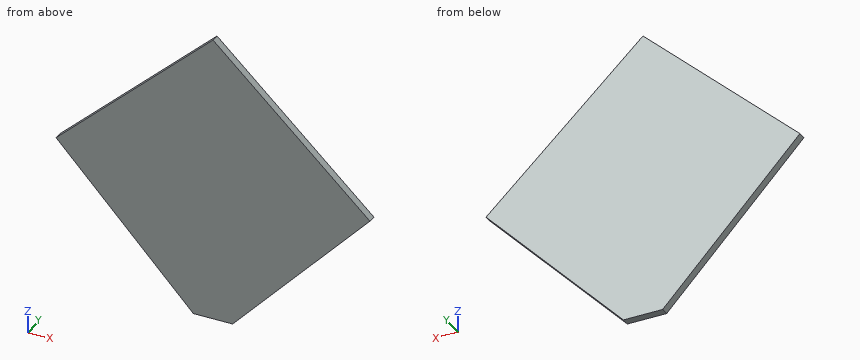
```python
from build123d import *

# Parameters (mm, degrees)
F1_DEPTH = 1


with BuildPart() as f1:
    # F0 (on Front) → F1 (new body)
    with BuildSketch(Plane.XZ):
        Polygon((-2.5, 0), (0, 0), (0, 18.5), (-20, 18.5), align=None)
        Polygon((0, 18.5), (0, 0), (2.5, 0), (20, 18.5), align=None)
        Polygon((-20, 18.5), (0, 18.5), (0, 37), align=None)
        Polygon((0, 37), (0, 18.5), (20, 18.5), align=None)
    extrude(amount=F1_DEPTH)


solid = f1.part
```
For this review, take the finished solid that the model builds, in its own axes (mm). Round coordinates to 2 decimals unless told otherwise and drop trailing zeros. Write each loop counter-clockwise with the first axis right and the second up, starting at its lowest first coordinate (ties: lowest second). Pieces come first, ordered by that corner, then holes. Notation, with made-up numbers: (10.25, 26.25) - (69.25, 26.25) arc R22 cw to (69.25, 58.25) - close; hole circle Ø8 at (80, -12.75). An arc over 180 degrees is marked (long way). Put each result on its own line as item: value.
Q1. Wall thickness on probe 1 along Z at (x, y) = (16, -0.45); probe 2 along Z at (x, y) = (-4, -0.5); probe 3 along X at (y, z) = (-0.5, 21.5): over which ranges is each line inside the solid? List them lowest first.
Solved:
probe 1: z = 14.27 to 22.2
probe 2: z = 1.59 to 33.3
probe 3: x = -16.76 to 16.76
Q2. We need section B-B (z = 12.5). Give the boundary of the cut face in (x, y), and give its area (3 significant figures).
Solved:
outline: (-14.32, -1) - (14.32, -1) - (14.32, 0) - (-14.32, 0) - close
area: 28.6 mm2
Q3. We need section C-C (x = 17). Give the boundary of the cut face in (y, z) (3 decimals).
Solved:
outline: (-1, 15.329) - (0, 15.329) - (0, 21.275) - (-1, 21.275) - close
Q4. We need section A-A (y = -0.3). Give the boundary of the cut face in (x, z).
Solved:
outline: (-20, 18.5) - (-2.5, 0) - (2.5, 0) - (20, 18.5) - (0, 37) - close
